Read the model definition and answer for the solid it produces. Units are mm, in the model's axes. Coordinates: 2 decimals unless noted, no trailing zeros. Order: outer loops, then holes, each group sorted by start corner. A loop starts at its lowest first (then second) coordinate and runs counter-clockwise, first axis right, second up. Notation, with made-up numbers: (46.5, 13) - (79.5, 13) arc R30 ccw to (79.5, 49) - close; hole circle Ø6 at (8, 54). An arc over 180 degrees is marked (long way). Write item = value, one per line.
from build123d import *

# Parameters (mm, degrees)
SKETCH1_W           = 20
SKETCH1_H           = 20
BOSS_EXTRUDE1_DEPTH = 400
SKETCH2_W           = 17
SKETCH2_H           = 17
CUT_EXTRUDE1_DEPTH  = 400
SKETCH3_R           = 2
CUT_EXTRUDE2_DEPTH  = 25
SKETCH4_R           = 2
CUT_EXTRUDE3_DEPTH  = 25
LPATTERN1_COUNT     = 3
LPATTERN1_PITCH     = 100


with BuildPart() as part:
    # Sketch1 → Boss-Extrude1 (new body)
    with BuildSketch(Plane.XY):
        Rectangle(SKETCH1_W, SKETCH1_H)
    extrude(amount=BOSS_EXTRUDE1_DEPTH)

    # Sketch2 → Cut-Extrude1 (cut)
    with BuildSketch(Plane(origin=(0, 0, 0), x_dir=(-1, 0, 0), z_dir=(0, 0, -1))):
        Rectangle(SKETCH2_W, SKETCH2_H)
    extrude(amount=-CUT_EXTRUDE1_DEPTH, mode=Mode.SUBTRACT)

    # Sketch3 → Cut-Extrude2 (cut)
    with BuildSketch(Plane(origin=(0, 10, 0), x_dir=(1, 0, 0), z_dir=(0, 1, 0))):
        with Locations((0, -75)):
            Circle(SKETCH3_R)
    cut_extrude2 = extrude(amount=-CUT_EXTRUDE2_DEPTH, mode=Mode.SUBTRACT)

    # Sketch4 → Cut-Extrude3 (cut)
    with BuildSketch(Plane(origin=(0, 10, 0), x_dir=(1, 0, 0), z_dir=(0, 1, 0))):
        with Locations((0, -115)):
            Circle(SKETCH4_R)
    cut_extrude3 = extrude(amount=-CUT_EXTRUDE3_DEPTH, mode=Mode.SUBTRACT)

    # LPattern1: Cut-Extrude2, Cut-Extrude3 ×3
    with Locations(*[(0, 0, i * LPATTERN1_PITCH) for i in range(1, LPATTERN1_COUNT)]):
        add(cut_extrude2, mode=Mode.SUBTRACT)
        add(cut_extrude3, mode=Mode.SUBTRACT)


solid = part.part
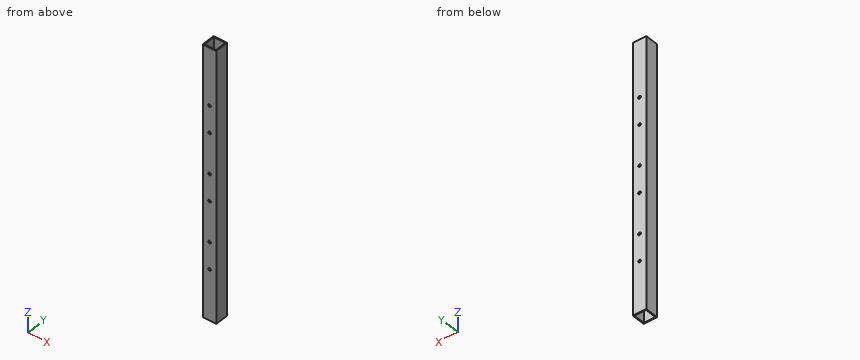
1) The part is cut by section A-A (y = -4). Determine the outline of the cut face in (x, z), and give its area (3 significant figures).
Returned:
outline = (-10, 0) - (-8.5, 0) - (-8.5, 400) - (-10, 400) - close; (8.5, 0) - (10, 0) - (10, 400) - (8.5, 400) - close
area = 1,200 mm^2
2) Straight lines are drawn through the part: line 1 along X through (y, z) = (-7.75, 113); line 2 along X through (y, z) = (9.45, 115). For each, find the intervals that lie inside material, in ascending order. Write a range as from..to.
Returned:
line_1 = -10..-8.5, 8.5..10
line_2 = -10..-2, 2..10
3) A flat-ended cylindrical pin translates along its axis: pin 1 Ø3 at (x, z) = (0, 275) entering from +Y. Find the tip coordinate at first contact, or state that the pin passes through.
Returned:
pin_1 = through
4) The part is cut by section B-B (z = 356.5). Determine the outline of the cut face in (x, y).
Returned:
outline = (-10, -10) - (10, -10) - (10, 10) - (-10, 10) - close; hole (-8.5, -8.5) - (8.5, -8.5) - (8.5, 8.5) - (-8.5, 8.5) - close
